from build123d import *

# Parameters (mm, degrees)
SKETCH1_R           = 2.7686
SKETCH1_R_2         = 1.016
BOSS_EXTRUDE1_DEPTH = 1.8034
FILLET1_R           = 0.381
CHAMFER1_SIZE       = 0.381


with BuildPart() as part:
    # Sketch1 → Boss-Extrude1 (new body)
    with BuildSketch(Plane(origin=(0, 0, 0), x_dir=(1, 0, 0), z_dir=(0, 1, 0))):
        with Locations(Location((0, 0, 0), (0, 0, 270))):
            Circle(SKETCH1_R)
        with Locations(Location((0, 0, 0), (0, 0, 270))):
            Circle(SKETCH1_R_2, mode=Mode.SUBTRACT)
    extrude(amount=BOSS_EXTRUDE1_DEPTH)

    # Fillet1
    fillet1_edges = [part.edges().sort_by_distance(p)[0] for p in [
        (0, 0, -2.7686),
        (0, 1.8034, -2.7686),
    ]]
    fillet(fillet1_edges, radius=FILLET1_R)

    # Chamfer1
    chamfer1_edges = [part.edges().sort_by_distance(p)[0] for p in [
        (0, 0, -1.016),
        (0, 1.8034, -1.016),
    ]]
    chamfer(chamfer1_edges, length=CHAMFER1_SIZE)


solid = part.part
The listing builds one solid part. Answer for the finished solid, in the listing's coordinates (mm). Round coordinates to 2 decimals unless told otherwise and drop trailing zeros. Write each loop counter-clockwise with the first axis right and the second up, starting at its lowest first coordinate (ties: lowest second). Pieces come first, ordered by that corner, then holes. Notation, with made-up numbers: M -9.75,73.5 L 16.25,73.5 A25 cw 16.25,96.5 Z; hole C 75.25,-35.75 d2. An arc over 180 degrees is marked long. Write each question's results on one line, items separated by ' | '. Start each with the question number.
Item 1: Find section C-C on y = 0.9. Write down the section's boundary in (x, z), and give its area (3 significant figures).
Item 2: Find section B-B on x = 0. Write down the section's boundary in (y, z), and give its area (3 significant figures).
Item 3: Find section A-A on z = 0. Write down the section's boundary in (x, y), and give its area (3 significant figures).
Item 4: The mould has two halves that part along Z. Classify faces 1 (the cylindrical face through (-0.99, 0.89, -0.22)), 2 (the flat face through (-2, 1.803, 0)), 3 (the cylindrical face through (-1.06, 0.894, 2.557)): +Z half, -Z half, draft (parallel to the pull), parting line (faces both ways), or undercut.
Item 5: Straight lines are drawn through the part: probe 1 along X at (y, z) = (1.2, 0); probe 2 along Z at (x, y) = (1.4, 0.65); probe 3 along Z at (x, y) = (-0.1, 1.4). For each, find the intervals that lie inside material, in ascending order.
Item 6: Given pin 1 Ø2.5 at (x, z) = (0, 0) entering from -Y, flat-ended and moving along its own axis, determine where the tip first touches the part or whether it passes through.
Answer block:
1) outline: C 0,0 d5.54; hole C 0,0 d2.03 | area: 20.8 mm²
2) outline: M 0,-2.39 A0.38 ccw 0.38,-2.77 L 1.42,-2.77 A0.38 ccw 1.8,-2.39 L 1.8,-1.4 L 1.42,-1.02 L 0.38,-1.02 L 0,-1.4 Z; M 0,1.4 L 0.38,1.02 L 1.42,1.02 L 1.8,1.4 L 1.8,2.39 A0.38 ccw 1.42,2.77 L 0.38,2.77 A0.38 ccw 0,2.39 Z | area: 5.91 mm²
3) outline: M -2.77,0.38 A0.38 ccw -2.39,0 L -1.4,0 L -1.02,0.38 L -1.02,1.42 L -1.4,1.8 L -2.39,1.8 A0.38 ccw -2.77,1.42 Z; M 1.02,0.38 L 1.4,0 L 2.39,0 A0.38 ccw 2.77,0.38 L 2.77,1.42 A0.38 ccw 2.39,1.8 L 1.4,1.8 L 1.02,1.42 Z | area: 5.91 mm²
4) face 1: undercut | face 2: draft | face 3: parting line
5) probe 1: x = -2.77 to -1.02, 1.02 to 2.77 | probe 2: z = -2.39 to 2.39 | probe 3: z = -2.77 to -1.01, 1.01 to 2.77
6) pin 1: stops at y = 0.15
